Build history of the part. All positions in model axes, mm. A direction names the side the tool comes from. Coordinates: 2 decimals unless noted, no trailing zeros. Order: outer loops, then holes, each group sorted by start corner. A loop starts at its lowest first (then second) coordinate and runs counter-clockwise, first axis right, second up. Notation, with made-up numbers: (-18.75, 83.25) - (1.25, 83.25) arc R20 cw to (1.25, 108.25) - close; hole circle Ø3 at (55, 60.25). An arc over 180 degrees is marked (long way). One line per item, written item: value.
from build123d import *

# Parameters (mm, degrees)
SKETCH1_W            = 30
SKETCH1_H            = 48.5
SKETCH1_R            = 1.55
BOSS_EXTRUDE1_DEPTH  = 15
SKETCH1_3_R          = 6.5
CUT_EXTRUDE2_DEPTH   = 2
CUT_EXTRUDE3_DEPTH   = 4.5
BOSS_EXTRUDE2_DEPTH  = 15
CUT_EXTRUDE4_DEPTH   = 11
SKETCH2_5_R          = 1.6
BOSS_EXTRUDE4_DEPTH  = 13
SKETCH2_6_R          = 1.6
CUT_EXTRUDE5_DEPTH   = 2
CUT_EXTRUDE6_DEPTH   = 11
BOSS_EXTRUDE8_DEPTH  = 4
BOSS_EXTRUDE10_DEPTH = 4
CUT_EXTRUDE8_DEPTH   = 2
CUT_EXTRUDE9_REACH   = 17
FILLET1_R            = 1.5


with BuildPart() as part:
    # Sketch1 → Boss-Extrude1 (new body)
    with BuildSketch(Plane.XY):
        with Locations((15, 20.25)):
            Rectangle(SKETCH1_W, SKETCH1_H)
        with Locations((5, 40.95)):
            Circle(SKETCH1_R, mode=Mode.SUBTRACT)
        with Locations((25, 40.95)):
            Circle(SKETCH1_R, mode=Mode.SUBTRACT)
    extrude(amount=BOSS_EXTRUDE1_DEPTH)

    # Sketch1<3> → Cut-Extrude2 (cut)
    with BuildSketch(Plane.XY):
        with Locations((15, 8)):
            Circle(SKETCH1_3_R)
    extrude(amount=CUT_EXTRUDE2_DEPTH, mode=Mode.SUBTRACT)

    # Sketch4 → Cut-Extrude3 (cut)
    with BuildSketch(Plane.XY.offset(15)):
        Polygon((8.233161507, 40.95), (6.616580754, 43.75), (3.383419246, 43.75), (1.766838493, 40.95), (3.383419246, 38.15), (6.616580754, 38.15), align=None)
        Polygon((28.233161507, 40.95), (26.616580754, 43.75), (23.383419246, 43.75), (21.766838493, 40.95), (23.383419246, 38.15), (26.616580754, 38.15), align=None)
    extrude(amount=-CUT_EXTRUDE3_DEPTH, mode=Mode.SUBTRACT)

    # Sketch2 → Boss-Extrude2 (add)
    with BuildSketch(Plane.XY):
        Polygon((-25.480933218, 164.5), (18.195494894, 44.5), (30, 44.5), (-13.676428112, 164.5), (-16.868961429, 164.5), align=None)
        Polygon((-32.092545942, 164.5), (-38.704158666, 164.5), (4.972269446, 44.5), (18.195494894, 44.5), (-25.480933218, 164.5), align=None)
        Polygon((-47.316130455, 164.5), (0, 34.5), (0, 44.5), (4.972269446, 44.5), (-38.704158666, 164.5), align=None)
        Polygon((-3.192533317, 34.5), (0, 34.5), (-47.316130455, 164.5), (-50.508663772, 164.5), align=None)
        Polygon((0, 25.7285868), (0, 34.5), (-3.192533317, 34.5), align=None)
    extrude(amount=BOSS_EXTRUDE2_DEPTH)

    # Sketch2<3> → Cut-Extrude4 (cut)
    with BuildSketch(Plane.XY):
        Polygon((-32.092545942, 164.5), (-38.704158666, 164.5), (4.972269446, 44.5), (18.195494894, 44.5), (-25.480933218, 164.5), align=None)
        Polygon((-41.433935423, 172), (-38.704158666, 164.5), (-32.092545942, 164.5), (-34.822322699, 172), align=None)
        Polygon((-37.552099456, 179.5), (-44.16371218, 179.5), (-42.022322699, 173.616580754), (-41.433935423, 172), (-34.822322699, 172), align=None)
        Polygon((-30.940486732, 179.5), (-37.552099456, 179.5), (-34.822322699, 172), (-28.210709975, 172), align=None)
        Polygon((-34.822322699, 172), (-32.092545942, 164.5), (-25.480933218, 164.5), (-27.622322699, 170.383419246), (-28.210709975, 172), align=None)
    extrude(amount=CUT_EXTRUDE4_DEPTH, mode=Mode.SUBTRACT)

    # Sketch2<5> → Boss-Extrude4 (add)
    with BuildSketch(Plane.XY):
        Polygon((-52.775683969, 179.5), (-47.316130455, 164.5), (-16.868961429, 164.5), (-22.328514943, 179.5), align=None)
        with Locations((-44.822322699, 172)):
            Circle(SKETCH2_5_R, mode=Mode.SUBTRACT)
        with Locations((-24.822322699, 172)):
            Circle(SKETCH2_5_R, mode=Mode.SUBTRACT)
    extrude(amount=BOSS_EXTRUDE4_DEPTH)

    # Sketch2<6> → Cut-Extrude5 (cut)
    with BuildSketch(Plane.XY):
        Polygon((-52.775683969, 179.5), (-47.316130455, 164.5), (-16.868961429, 164.5), (-22.328514943, 179.5), align=None)
        with Locations((-44.822322699, 172)):
            Circle(SKETCH2_6_R, mode=Mode.SUBTRACT)
        with Locations((-24.822322699, 172)):
            Circle(SKETCH2_6_R, mode=Mode.SUBTRACT)
    extrude(amount=CUT_EXTRUDE5_DEPTH, mode=Mode.SUBTRACT)

    # Sketch2<7> → Cut-Extrude6 (cut)
    with BuildSketch(Plane.XY):
        Polygon((-37.552099456, 179.5), (-44.16371218, 179.5), (-42.022322699, 173.616580754), (-41.433935423, 172), (-34.822322699, 172), align=None)
        Polygon((-41.433935423, 172), (-38.704158666, 164.5), (-32.092545942, 164.5), (-34.822322699, 172), align=None)
        Polygon((-34.822322699, 172), (-32.092545942, 164.5), (-25.480933218, 164.5), (-27.622322699, 170.383419246), (-28.210709975, 172), align=None)
        Polygon((-30.940486732, 179.5), (-37.552099456, 179.5), (-34.822322699, 172), (-28.210709975, 172), align=None)
    extrude(amount=CUT_EXTRUDE6_DEPTH, mode=Mode.SUBTRACT)

    # Sketch2<9> → Boss-Extrude8 (add)
    with BuildSketch(Plane.XY):
        Polygon((-32.092545942, 164.5), (-38.704158666, 164.5), (4.972269446, 44.5), (18.195494894, 44.5), (-25.480933218, 164.5), align=None)
    extrude(amount=BOSS_EXTRUDE8_DEPTH)

    # Sketch2<11> → Boss-Extrude10 (add)
    with BuildSketch(Plane.XY):
        Polygon((-41.433935423, 172), (-38.704158666, 164.5), (-32.092545942, 164.5), (-34.822322699, 172), align=None)
        Polygon((-37.552099456, 179.5), (-44.16371218, 179.5), (-42.022322699, 173.616580754), (-41.433935423, 172), (-34.822322699, 172), align=None)
        Polygon((-34.822322699, 172), (-32.092545942, 164.5), (-25.480933218, 164.5), (-27.622322699, 170.383419246), (-28.210709975, 172), align=None)
        Polygon((-30.940486732, 179.5), (-37.552099456, 179.5), (-34.822322699, 172), (-28.210709975, 172), align=None)
    extrude(amount=BOSS_EXTRUDE10_DEPTH)

    # Sketch2<12> → Cut-Extrude8 (cut)
    with BuildSketch(Plane.XY):
        Polygon((-37.552099456, 179.5), (-44.16371218, 179.5), (-42.022322699, 173.616580754), (-41.433935423, 172), (-34.822322699, 172), align=None)
        Polygon((-41.433935423, 172), (-38.704158666, 164.5), (-32.092545942, 164.5), (-34.822322699, 172), align=None)
        Polygon((-34.822322699, 172), (-32.092545942, 164.5), (-25.480933218, 164.5), (-27.622322699, 170.383419246), (-28.210709975, 172), align=None)
        Polygon((-30.940486732, 179.5), (-37.552099456, 179.5), (-34.822322699, 172), (-28.210709975, 172), align=None)
    extrude(amount=CUT_EXTRUDE8_DEPTH, mode=Mode.SUBTRACT)

    # Sketch6 → Cut-Extrude9 (cut, up to next)
    with BuildSketch(Plane(origin=(0, 0, 0), x_dir=(-1, 0, 0), z_dir=(0, 0, -1)), mode=Mode.PRIVATE) as cut_extrude9_sk1:
        Polygon((-18.195494894, 44.5), (-4.972269446, 44.5), (0.487284068, 59.5), (-12.73594138, 59.5), align=None)
    cut_extrude9_tool1 = extrude(cut_extrude9_sk1.sketch, amount=-CUT_EXTRUDE9_REACH, mode=Mode.PRIVATE) & part.part
    add(cut_extrude9_tool1.solids().sort_by_distance((8.854105, 52, 0))[0], mode=Mode.SUBTRACT)

    # Fillet1
    fillet1_edges = [part.edges().sort_by_distance(p)[0] for p in [
        (-25.254331886, 95.1142934, 0),
        (8.161785944, 104.5, 0),
        (-25.254331886, 95.1142934, 15),
        (8.161785944, 104.5, 15),
    ]]
    fillet(fillet1_edges, radius=FILLET1_R)


solid = part.part
1. Band-saw the part on A-A, the plane y = 8. Give the cut face in (x, z), and give its area (3 significant figures).
Values found:
outline: (0, 0) - (8.5, 0) - (8.5, 2) - (21.5, 2) - (21.5, 0) - (30, 0) - (30, 15) - (0, 15) - close
area: 424 mm2
2. Probe line 1 along X through (y, z) = (172, 8.5); line 2 along Z through (x, y) = (-32, 167); line 3 along Z through (x, y) = (-15, 131). List the from-to ranges inside material, lowest first.
Values found:
line 1: x = -50.05 to -46.42, -43.22 to -41.43, -28.21 to -26.42, -23.22 to -19.6
line 2: z = 2 to 4, 11 to 13
line 3: z = 0 to 4, 11 to 15
3. Flat gauge pins, fed straight in: P1, Ø1.9, axis at x = 5, y = 40.95, coming from the -Z side; P2, Ø4, axis at y = 21.5, z = 4, coming from the -X side; P3, Ø8, axis at y = 106.5, z = 10, coming from the -X side; P4, Ø4, axis at x = -24.82, y = 172, coming from the -Z side. Where does each tip first touch, or does it go through?
Values found:
P1: passes through
P2: stops at x = 0
P3: stops at x = -30.85
P4: stops at z = 2
4. 3-axis set-ups, long thin cutter, end or side, ignore diameter. For faces 1 (the face through (25, 38.15, 13)), 2 (the face through (-35, 172, 13)), 3 (the face through (8.506, 8.286, 0.986)): which of +Z, -Z, +X, -X, +Y, -Y reach the whole face in a straight line?
Values found:
face 1: +Z
face 2: +Z, +X, -X, +Y
face 3: -Z
5. Two-plate mould, pull along Z, no slides. Class faces 4 (the face through (6.4, 42.2, 10.5)), 5 (the face through (-13, 112, 11)), 6 (the face through (-24.084, 170.581, 7.423)): pulls with the +Z half, pulls with the -Z half, needs draft (parallel to the pull), parting line crosses it, or undercut.
Values found:
face 4: pulls with the +Z half
face 5: undercut
face 6: needs draft
